Source: CAD feature listing. Evaluate the final solid. Frame: model axes, mm. Coordinates: 2 decimals unless noted, no trailing zeros. Loops run counter-clockwise (first coordinate to the right, second up) from the corner with the lowest first, then second, coordinate; pieces in that order, holes last.
from build123d import *

# Parameters (mm, degrees)
F0_W     = 1219.2
F0_H     = 2438.4
F0_W_2   = 203.2
F0_H_2   = 304.8
F1_DEPTH = 3.175


with BuildPart() as f1:
    # F0 (on Front) → F1 (new body, symmetric)
    with BuildSketch(Plane.XZ):
        Rectangle(F0_W, F0_H)
        with Locations((11.608229, -20.958262)):
            Rectangle(F0_W_2, F0_H_2, mode=Mode.SUBTRACT)
        with Locations((11.608229, 446.332766)):
            Rectangle(F0_W_2, F0_H_2, mode=Mode.SUBTRACT)
    extrude(amount=F1_DEPTH, both=True)


solid = f1.part
Q1. Section B-B, the plane x = 68. Return the cut outline in (y, z) (3 decimals).
Q2. Section A-A, the plane z = 463. Return the cut outline in (x, y) (3 decimals), plus the area to 3 significant figures.
Q3. Line query: line 1 along Z through (x, y) = (31, 3); line 2 along X through (y, z) = (2, -127). Output: solid intervals per line, ascending.
Q4. Section C-C, the plane y = -1. Return the cut outline in (x, z).
Derived:
1. outline: (-3.175, -1219.2) - (3.175, -1219.2) - (3.175, -173.358) - (-3.175, -173.358) - close; (-3.175, 131.442) - (3.175, 131.442) - (3.175, 293.933) - (-3.175, 293.933) - close; (-3.175, 598.733) - (3.175, 598.733) - (3.175, 1219.2) - (-3.175, 1219.2) - close
2. outline: (-609.6, -3.175) - (-89.992, -3.175) - (-89.992, 3.175) - (-609.6, 3.175) - close; (113.208, -3.175) - (609.6, -3.175) - (609.6, 3.175) - (113.208, 3.175) - close
2. area: 6,450 mm2
3. line 1: z = -1219.2 to -173.36, 131.44 to 293.93, 598.73 to 1219.2
3. line 2: x = -609.6 to -89.99, 113.21 to 609.6
4. outline: (-609.6, -1219.2) - (609.6, -1219.2) - (609.6, 1219.2) - (-609.6, 1219.2) - close; hole (-89.99, -173.36) - (113.21, -173.36) - (113.21, 131.44) - (-89.99, 131.44) - close; hole (-89.99, 293.93) - (113.21, 293.93) - (113.21, 598.73) - (-89.99, 598.73) - close
